Input: part model. Units: mm. Frame: model coordinates. A direction names the side the tool comes from. Give positions to 0.01 mm unless a question says otherwise; leave off trailing zeros. Order: outer loops, then holes, each group sorted by start corner. A loop starts at its lowest first (then second) coordinate and runs counter-clockwise, first axis right, second up. Notation, with made-up numbers: (80, 45.5) - (95, 45.5) arc R30 ccw to (95, 70.5) - close; hole circle Ø7 at (-38, 59). An arc over 180 degrees is marked (long way). Answer in a Markdown table with one row per item. Add a question column.
1. Access query for faces 4 (the face through (7, 0, 49)), 5 (the face through (7, -2, 49)). Directions: +Z, -Z, +X, -X, +Y, -Y. A direction counts if a zero-diameter tool reaches every point of the face in a straight line with its end or side. Return the directions, or none.
2. Section query D-D on z = 80. Return loops of the section in (x, y).
3. Mould query, pull axis Z, two halves, no side actions, for faces 1 (the face through (14.01, -9.06, 25.35)), 2 (the face through (13, -9, 49)), 3 (the face through (10, -1, 100)). Classes: released by +Z, released by -Z, zero draft, split by the parting line, or undercut.
4. Section query A-A on x = 6.52. Return loops of the section in (y, z).
5. Section query C-C on y = -7.5. Return loops of the section in (x, z), and give its area (3 significant figures).
6. Ray query, line 1 (Z direction, x = 3.5, y = -0.95) (3 decimals); line 2 (X direction, y = -0.7, z = 25); line 3 (Z direction, x = 3, y = -0.75). Return the intervals inside material, ascending. Write a range as [from, to].
7. Contact query for flat-ended pins moving along their axis: pin 1 (4 mm diameter, centred on x = 10.5, y = -3.5, fed in from +Z); pin 2 (2 mm diameter, centred on x = 6.52, z = 95, fed in from +Y); pin 3 (1 mm diameter, centred on x = 4, z = 19, fed in from -Y); pin 4 (6.5 mm diameter, centred on y = -7.5, z = 49.5, fed in from -X). Output: stop coordinate, or through.
8. Section query B-B on z = 25. Return loops of the section in (x, y).
```python
from build123d import *

# Parameters (mm, degrees)
EXTRUDE_1_DEPTH     = 100
SKETCH_4_R          = 1.6
CUT_EXTRUDE_3_DEPTH = 2
M3X0_5_1_D          = 2.5
M3X0_5_1_DEPTH      = 8.5
M3X0_5_1_TIP        = 0.751075774
SKETCH_2_R          = 1.6
CUT_EXTRUDE_4_DEPTH = 10


with BuildPart() as part:
    # ｽｹｯﾁ1 → ﾎﾞｽ - 押し出し1 (new body)
    with BuildSketch(Plane.XY):
        Polygon((0, 0), (15, 0), (15, -15), (13, -15), (13, -2), (0, -2), align=None)
    extrude(amount=EXTRUDE_1_DEPTH)

    # ｽｹｯﾁ4 → ｶｯﾄ - 押し出し3 (cut)
    with BuildSketch(Plane(origin=(0, 0, 0), x_dir=(1, 0, 0), z_dir=(0, 1, 0))):
        with Locations((3.5, -57.875)):
            Circle(SKETCH_4_R)
        with Locations((3.5, -42.125)):
            Circle(SKETCH_4_R)
    extrude(amount=-CUT_EXTRUDE_3_DEPTH, mode=Mode.SUBTRACT)

    # M3x0.5 ねじ穴1
    with Locations(Plane(origin=(6.52, 0, 75), x_dir=(0, 0, 1), z_dir=(0, 1, 0))):
        with Locations((0, 0), (-50, 0), (20, 0), (-70, 0)):
            Hole(M3X0_5_1_D / 2, depth=M3X0_5_1_DEPTH)
            with Locations((0, 0, -(M3X0_5_1_DEPTH + M3X0_5_1_TIP / 2))):  # 118° drill point
                Cone(0, M3X0_5_1_D / 2, M3X0_5_1_TIP, mode=Mode.SUBTRACT)

    # ｽｹｯﾁ2 → ｶｯﾄ - 押し出し4 (cut)
    with BuildSketch(Plane(origin=(15, 0, 0), x_dir=(0, 0, -1), z_dir=(1, 0, 0))):
        with Locations((-75, -7.5)):
            Circle(SKETCH_2_R)
        with Locations((-25, -7.5)):
            Circle(SKETCH_2_R)
    extrude(amount=-CUT_EXTRUDE_4_DEPTH, mode=Mode.SUBTRACT)


solid = part.part
```
Answer:
| question | item | result |
|---|---|---|
| 1 | face 4 | +Z, -Z, +X, -X, +Y |
| 1 | face 5 | +Z, -Z, -X, -Y |
| 2 | outline | (0, -2) - (13, -2) - (13, -15) - (15, -15) - (15, 0) - (0, 0) - close |
| 3 | face 1 | undercut |
| 3 | face 2 | zero draft |
| 3 | face 3 | released by +Z |
| 4 | outline | (-2, 0) - (0, 0) - (0, 3.75) - (-2, 3.75) - close; (-2, 6.25) - (0, 6.25) - (0, 23.75) - (-2, 23.75) - close; (-2, 26.25) - (0, 26.25) - (0, 73.75) - (-2, 73.75) - close; (-2, 76.25) - (0, 76.25) - (0, 93.75) - (-2, 93.75) - close; (-2, 96.25) - (0, 96.25) - (0, 100) - (-2, 100) - close |
| 5 | outline | (13, 0) - (15, 0) - (15, 23.4) - (13, 23.4) - close; (13, 26.6) - (15, 26.6) - (15, 73.4) - (13, 73.4) - close; (13, 76.6) - (15, 76.6) - (15, 100) - (13, 100) - close |
| 5 | area | 187 mm² |
| 6 | line 1 | z = [0, 40.525], [43.725, 56.275], [59.475, 100] |
| 6 | line 2 | x = [0, 5.27], [7.77, 15] |
| 6 | line 3 | z = [0, 40.61], [43.64, 56.36], [59.39, 100] |
| 7 | pin 1 | stops at z = 100 |
| 7 | pin 2 | passes through |
| 7 | pin 3 | stops at y = -2 |
| 7 | pin 4 | stops at x = 13 |
| 8 | outline | (0, -2) - (5.27, -2) - (5.27, 0) - (0, 0) - close; (7.77, -2) - (13, -2) - (13, -5.9) - (15, -5.9) - (15, 0) - (7.77, 0) - close; (13, -15) - (15, -15) - (15, -9.1) - (13, -9.1) - close |
